Read the model definition and answer for the solid it produces. Units are mm, in the model's axes. Face numbers are marked on the shaded views. A direction names the side the tool comes from. Coordinates: 2 decimals unless noted, no trailing zeros. Order: outer loops, then holes, each group sorted by start corner. A loop starts at its lowest first (then second) coordinate and runs counter-clockwise, first axis right, second up. Notation, with made-up numbers: (-34.5, -28.5) -> (-22.5, -28.5) arc R25 cw to (-22.5, -0.5) -> close; hole circle Ø4 at (-8, 52). An arc over 180 degrees is marked (long way). Answer as a JSON object with one key per item and string values. Group by question number.
1) Section B-B on x = 42.5 is taken. Determine the outline of the cut face in (y, z).
2) A tool of negligible diameter and unlimited length cuts with its end or side. For the marked faces 1, 2 and 3, from which of +Z, -Z, +X, -X, +Y, -Y can it reach the whole face along a straight path? Write none if from no direction.
3) Section C-C on z = 6 is taken. Determine the outline of the cut face in (x, y), and give its area (3 significant figures).
4) Section D-D on x = 7.5 is taken. Determine the outline of the cut face in (y, z), and give its area (3 significant figures).
5) Section A-A on y = 18.5 is taken. Determine the outline of the cut face in (x, z), and give its area (3 significant figures).
6) Consider L1, parallel to Y at x = 42.5, z = 10.25; L2, parallel to X at y = 22, z = 11.25; L3, parallel to X at y = 67, z = 6.5. Determine where each line is inside the solid, lowest interval first.
7) Given pin 1 (4.5 mm diameter, centred on x = 46, y = 67.5, fed in from -Z); pin 2 (1.5 mm diameter, centred on y = 70, z = 2.5, fed in from +X); pin 3 (1.5 mm diameter, centred on y = 40.5, z = 10, fed in from +X), each flat-ended and moving along its own axis, determine where each tip first touches the part or whether it passes through.
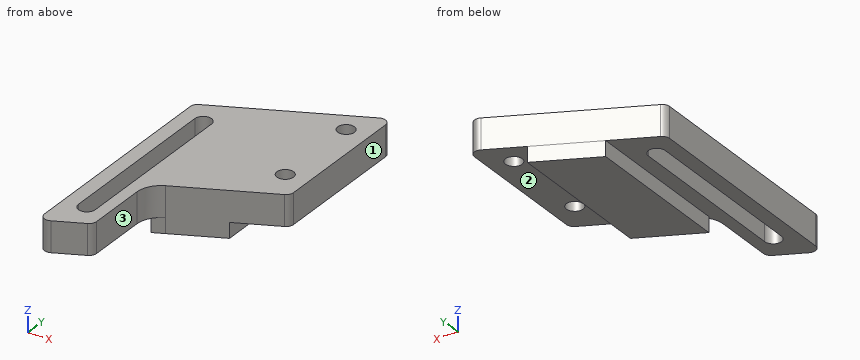
from build123d import *

# Parameters (mm, degrees)
BOSS_EXTRU_1_DEPTH      = 15
ESQUISSE4_OUTSIDE_W     = 74.658
ESQUISSE4_OUTSIDE_H     = 125.21
ENL_V_MAT_EXTRU_2_DEPTH = 5
ENL_V_MAT_EXTRU_3_DEPTH = 114.294624636
ENL_V_START             = -5
ENL_V_MAT_EXTRU_4_DEPTH = 5
CONG_1_R                = 2.5
D_GAGEMENT_M51_D        = 5.5


with BuildPart() as part:
    # Esquisse1 → Boss.-Extru.1 (new body)
    with BuildSketch(Plane.XY):
        Polygon((0, 0), (0, 77.236454327), (50, 100.551837235), (50, 23.315382908), align=None)
        with BuildLine():
            Line((4.75, 13.497307436), (4.75, 70.733761764))
            ThreePointArc((4.75, 70.733761764), (7.5, 73.483761764), (10.25, 70.733761764))
            Line((10.25, 70.733761764), (10.25, 13.497307436))
            ThreePointArc((10.25, 13.497307436), (7.5, 10.747307436), (4.75, 13.497307436))
        make_face(mode=Mode.SUBTRACT)
    extrude(amount=BOSS_EXTRU_1_DEPTH)

    # Esquisse4 outside → Enlèv. mat.-Extru.2 (cut)
    with BuildSketch(Plane(origin=(0, 0, 0), x_dir=(-1, 0, 0), z_dir=(0, 0, -1))):
        with Locations((-25, 50.276)):
            Rectangle(ESQUISSE4_OUTSIDE_W, ESQUISSE4_OUTSIDE_H)
        Polygon((-15.2, 84.324330731), (-15.2, 7.087876404), (-34.8, 16.227506504), (-34.8, 93.463960831), align=None, mode=Mode.SUBTRACT)
    extrude(amount=-ENL_V_MAT_EXTRU_2_DEPTH, mode=Mode.SUBTRACT)

    # Esquisse5 → Enlèv. mat.-Extru.3 (cut, through all)
    with BuildSketch(Plane.XY.offset(15)):
        with BuildLine():
            Line((50, 23.315382908), (50, 49.796452963))
            Line((50, 49.796452963), (18.819053906, 35.256539011))
            ThreePointArc((18.819053906, 35.256539011), (15.452868433, 32.304473581), (14.2, 28.006076714))
            Line((14.2, 28.006076714), (14.2, 6.621568746))
            Line((14.2, 6.621568746), (50, 23.315382908))
        make_face()
    extrude(amount=-ENL_V_MAT_EXTRU_3_DEPTH, mode=Mode.SUBTRACT)

    # Esquisse6 → Enlèv. mat.-Extru.4 (cut)
    with BuildSketch(Plane(origin=(0, 0, 0), x_dir=(-1, 0, 0), z_dir=(0, 0, -1)).offset(ENL_V_START)):
        with BuildLine():
            Line((-18.819053906, 35.256539011), (-15.2, 33.568946459))
            Line((-15.2, 33.568946459), (-15.2, 31.879060061))
            ThreePointArc((-15.2, 31.879060061), (-16.741717169, 33.854764476), (-18.819053906, 35.256539011))
        make_face()
    extrude(amount=ENL_V_MAT_EXTRU_4_DEPTH, mode=Mode.SUBTRACT)

    # Congé1
    cong_1_edges = [part.edges().sort_by_distance(p)[0] for p in [
        (0, 0, 10),
        (0, 77.236454327, 10),
        (50, 100.551837235, 10),
        (14.2, 6.621568746, 10),
        (50, 49.796452963, 10),
    ]]
    fillet(cong_1_edges, radius=CONG_1_R)

    # Dégagement M51 (through all)
    with Locations(Plane(origin=(42.5, 58.554529799, 15), x_dir=(1, 0, 0), z_dir=(0, 0, 1))):
        with Locations((0, 0), (0, 30)):
            Hole(D_GAGEMENT_M51_D / 2)


solid = part.part
Worked answers:
{
 "1": {"outline": "(46.3, 5) -> (55.8, 5) -> (55.8, 15) -> (46.3, 15) -> close; (61.3, 5) -> (85.8, 5) -> (85.8, 15) -> (61.3, 15) -> close; (91.3, 5) -> (97.05, 5) -> (97.05, 15) -> (91.3, 15) -> close"},
 "2": {"face 1": "+Z, -Z, +X, +Y, -Y", "face 2": "-Z, +X, +Y, -Y", "face 3": "+Z, -Z, +X, -Y"},
 "3": {"outline": "(0, 3.92) arc R2.5 ccw to (3.56, 1.66) -> (12.76, 5.95) arc R2.5 ccw to (14.2, 8.21) -> (14.2, 28.01) arc R8 cw to (18.82, 35.26) -> (48.56, 49.12) arc R2.5 ccw to (50, 51.39) -> (50, 96.63) arc R2.5 ccw to (46.44, 98.89) -> (1.44, 77.91) arc R2.5 ccw to (0, 75.64) -> close; hole (4.75, 13.5) arc R2.75 ccw to (10.25, 13.5) -> (10.25, 70.73) arc R2.75 ccw to (4.75, 70.73) -> close; hole circle Ø5.5 at (42.5, 58.55); hole circle Ø5.5 at (42.5, 88.55)", "area": "2,520 mm²"},
 "4": {"outline": "(3.5, 5) -> (10.75, 5) -> (10.75, 15) -> (3.5, 15) -> close; (73.48, 5) -> (80.73, 5) -> (80.73, 15) -> (73.48, 15) -> close", "area": "145 mm²"},
 "5": {"outline": "(0, 5) -> (4.75, 5) -> (4.75, 15) -> (0, 15) -> close; (10.25, 5) -> (14.2, 5) -> (14.2, 15) -> (10.25, 15) -> close", "area": "87.0 mm²"},
 "6": {"L1": "y = 46.3 to 55.8, 61.3 to 85.8, 91.3 to 97.05", "L2": "x = 0 to 4.75, 10.25 to 14.2", "L3": "x = 0 to 4.75, 10.25 to 50"},
 "7": {"pin 1": "stops at z = 5", "pin 2": "stops at x = 34.8", "pin 3": "stops at x = 31.67"}
}
